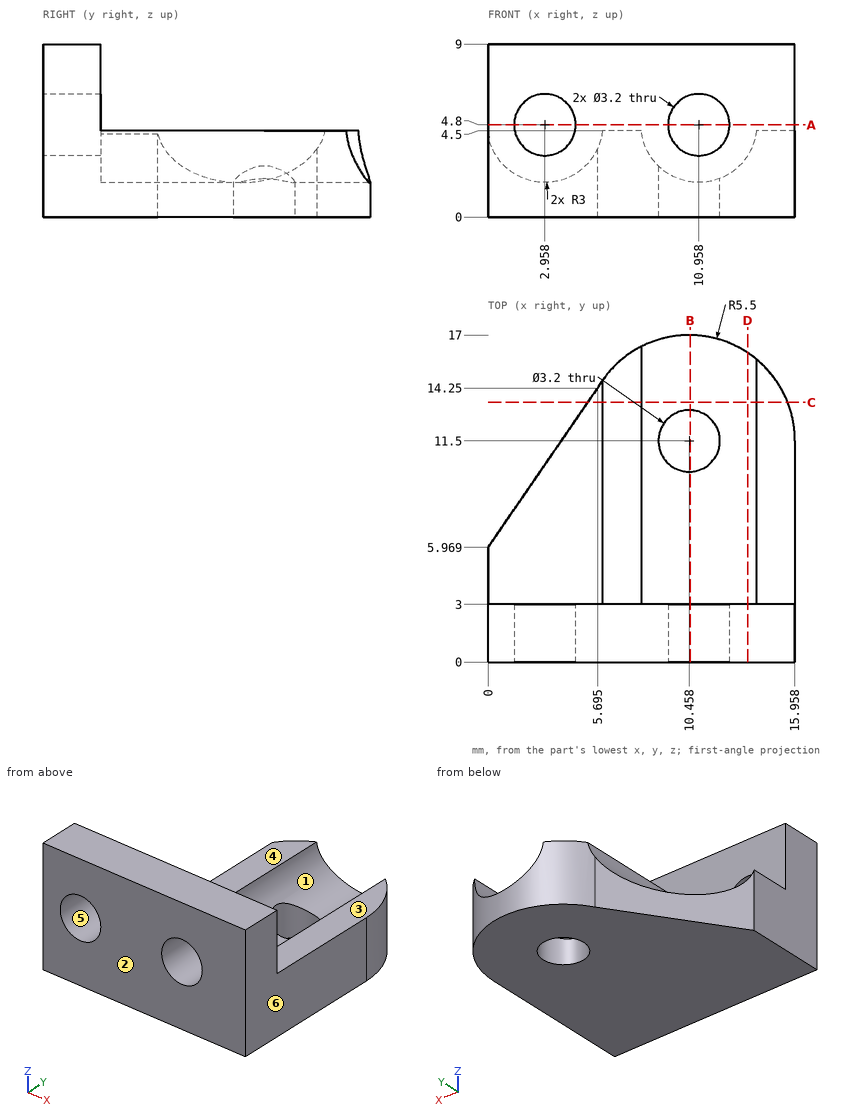
The drawing under review shows one solid part. Ordinate dimensions are in mm from its lowest x, y, z. A direction names the side the tool comes from. Round coordinates to 2 decimals unless told otherwise and drop trailing zeros. Loops run counter-clockwise (first coordinate to the right, second up) from the corner with the lowest first, then second, coordinate; pieces in that order, holes last. Notation, with made-up numbers: (6.25, -14.75) - (56.25, -14.75) arc R5 ccw to (56.25, -7.75) - close; hole circle Ø10 at (71.25, 68.5). An arc over 180 degrees is marked (long way). Use one line per item in the form item = value.
Item 1: Clearance check with flat-ended pins moving along their axes: P1, Ø0.6, axis at x = 14.5, y = 7.5, coming from the +Z side; P2, Ø1.9, axis at x = 10.958, z = 4.8, coming from the +Y side; P3, Ø2, axis at x = 7, z = 1.5, coming from the +Y side. State where each tip first meets the part, or that it passes through.
Answers:
P1 = 4.5
P2 = through
P3 = 16.42
Item 2: Tool access review of the marked faces 1, 2 and 3: name each direction out of +Z, -Z, +X, -X, +Y, -Y from which nothing blocks a thin tool from reaching the whole face with its end or side.
Answers:
face_1 = +Z, +Y
face_2 = +Z, -Z, +X, -X, -Y
face_3 = +Z, +X, -X, +Y
Item 3: Consider section A-A on z = 4.8. Write out the cut boundary in (x, y), then the cut area to 3 significant figures.
Answers:
outline = (0, 0) - (1.36, 0) - (1.36, 3) - (0, 3) - close; (4.56, 0) - (9.36, 0) - (9.36, 3) - (4.56, 3) - close; (12.56, 0) - (15.96, 0) - (15.96, 3) - (12.56, 3) - close
area = 28.7 mm^2
Item 4: Consider section D-D on x = 13.5. Write out the cut boundary in (y, z).
Answers:
outline = (0, 0) - (16.08, 0) - (16.08, 3.21) - (3, 3.21) - (3, 9) - (0, 9) - close
Item 5: Mouldability with a two-part tool opening along Z and no side actions: class the marked faces 4, 5 and 6 as +Z half, -Z half, draft (parallel to the pull), parting line (faces both ways), or undercut.
Answers:
face_4 = +Z half
face_5 = undercut
face_6 = draft
Item 6: Consider section C-C on y = 13.5. Write out the cut boundary in (x, z).
Answers:
outline = (5.18, 0) - (15.58, 0) - (15.58, 4.5) - (13.94, 4.5) arc R3 cw to (7.97, 4.5) - (5.94, 4.5) arc R3 cw to (5.18, 2.78) - close
Item 7: Consider section B-B on x = 10.5. Write out the cut boundary in (y, z) (1 decimal).
Answers:
outline = (0, 0) - (9.9, 0) - (9.9, 1.8) - (3, 1.8) - (3, 3.3) - (0, 3.3) - close; (0, 6.3) - (3, 6.3) - (3, 9) - (0, 9) - close; (13.1, 0) - (17, 0) - (17, 1.8) - (13.1, 1.8) - close
Item 8: For line 1 (Z direction, x = 7.5, y = 12.75); line 2 (Y direction, x = 8, z = 6.75); line 3 (X direction, y = 11.5, z = 1.2), list the stretches that pass through material, from the lowest coordinate up.
Answers:
line_1 = 0 to 4.5
line_2 = 0 to 3
line_3 = 3.8 to 8.86, 12.06 to 15.96
